Source: CAD feature listing. Evaluate the final solid. Frame: model axes, mm. A direction names the side the tool comes from. Give positions to 0.01 mm unless a question says otherwise; leave off trailing zeros. Write each loop counter-clockwise with the first axis right and the second up, starting at its lowest first coordinate (ties: lowest second). Pieces come first, ordered by that corner, then holes. Notation, with made-up numbers: (52, 42) -> (88, 42) arc R21 cw to (88, 56) -> close; hole circle Ø1 at (43, 53.25). An arc over 180 degrees is marked (long way). Use a Markdown table: item, result. Add a question column.
Autodesk Inventor part; units mm, degrees
ref_plane "YZ Plane" through (0, 0, 0) normal (1, 0, 0) x (0, 1, 0)
ref_plane "XZ Plane" through (0, 0, 0) normal (0, 1, 0) x (-1, 0, 0)
ref_plane "XY Plane" through (0, 0, 0) normal (0, 0, 1) x (1, 0, 0)
sketch "Sketch1" plane through (0, 0, 0) normal (0, 0, 1) x (1, 0, 0)
  circle A0 centre (-25.4186, 8.5236) radius 12.7
  dimension "d0" = 25.4
extrude "Extrusion1" add sketch "Sketch1" along normal blind 6.35
sketch "Sketch2" plane through (-25.4186, 8.5236, 6.35) normal (0, 0, 1) x (1, 0, 0)
  circle A0 centre (0, 0) radius 12.7
  circle A1 centre (0, 0) radius 7.9375
  dimension "d3" = 15.875
extrude "Extrusion2" add sketch "Sketch2" along normal blind 12.7 contours A1
sketch "Sketch3" plane through (-25.4186, 8.5236, 19.05) normal (0, 0, 1) x (1, 0, 0)
  circle A0 centre (0, 0) radius 7.9375
  circle A1 centre (0, 0) radius 3.175
  dimension "d6" = 6.35
extrude "Extrusion3" add sketch "Sketch3" along normal blind 44.45 contours A1
thread "Thread1"
chamfer "Chamfer1" distance 0.381 angle 45 1 edges at (-28.5936, 8.5236, 63.5)
properties part number "PP-00012"
(1) Cut plane B-B on x = -21.5. Return the cut outline in (y, z), then the cut area to 3 significant figures.
(2) Cut plane C-C on z = 5. Return the cut outline in (x, y), then the cut area to 3 significant figures.
(3) Cut plane A-A on y = 13. Return the cut outline in (x, z), then the cut area to 3 significant figures.
(4) First-contact query: pin 1 Ø7.5 at (x, y) = (-31, 12.5) entering from +Z; pin 2 Ø1.5 at (y, z) = (4, 31) entering from -X; pin 3 Ø10 at (y, z) = (14.5, 29) entering from -X; pin 4 Ø12 at (x, z) = (-18.5, 45) entering from -Y. Flat tips, straight axial feed; report the tip coordinate or a pass-through.
(5) Cut plane D-D on x = -16.25. Return the cut outline in (y, z), then the cut area to 3 significant figures.
(6) Access query for faces 1 (the cylindrical face through (-22.486, 9.74, 40.776)), 2 (the flat face through (-25, 9, 63.5)). Directions: +Z, -Z, +X, -X, +Y, -Y. A direction counts if a zero-diameter tool reaches every point of the face in a straight line with its end or side. Return the directions, or none.
(7) Material intervals for L1, parallel to Z at x = -30, y = -0.25; L2, parallel to Z at x = -29, y = 2; L3, parallel to Y at x = -30, z = 13, sorted ascending.
Output:
| question | item | result |
|---|---|---|
| 1 | outline | (-3.56, 0) -> (20.6, 0) -> (20.6, 6.35) -> (15.43, 6.35) -> (15.43, 19.05) -> (1.62, 19.05) -> (1.62, 6.35) -> (-3.56, 6.35) -> close |
| 1 | area | 329 mm^2 |
| 2 | outline | circle Ø25.4 at (-25.42, 8.52) |
| 2 | area | 507 mm^2 |
| 3 | outline | (-37.3, 0) -> (-13.53, 0) -> (-13.53, 6.35) -> (-18.86, 6.35) -> (-18.86, 19.05) -> (-31.97, 19.05) -> (-31.97, 6.35) -> (-37.3, 6.35) -> close |
| 3 | area | 317 mm^2 |
| 4 | pin 1 | z = 63.19 |
| 4 | pin 2 | through |
| 4 | pin 3 | x = -28.44 |
| 4 | pin 4 | y = 5.48 |
| 5 | outline | (-0.26, 0) -> (17.31, 0) -> (17.31, 6.35) -> (-0.26, 6.35) -> close |
| 5 | area | 112 mm^2 |
| 6 | face 1 | +Z |
| 6 | face 2 | +Z, +X, -X, +Y, -Y |
| 7 | L1 | 0 to 6.35 |
| 7 | L2 | 0 to 19.05 |
| 7 | L3 | 2.04 to 15.01 |
